The model under review builds one solid part; all positions refer to its coordinate system, in mm. Give positions to 0.01 mm unless a question says otherwise; leave off trailing zeros. Order: outer loops, then holes, each group sorted by start corner. A loop starts at its lowest first (then second) coordinate and runs counter-clockwise, first axis right, second up. Notation, with made-up numbers: (66.25, -26.75) -> (115.25, -26.75) arc R35 ccw to (115.25, 11.25) -> close; hole circle Ø1 at (58.5, 16.25). An arc over 180 degrees is marked (long way). Answer as a JSON object with one key per item and string values. Group by question number.
Autodesk Inventor part; units mm, degrees
ref_plane "YZ Plane" through (0, 0, 0) normal (1, 0, 0) x (0, 1, 0)
ref_plane "XZ Plane" through (0, 0, 0) normal (0, 1, 0) x (-1, 0, 0)
ref_plane "XY Plane" through (0, 0, 0) normal (0, 0, 1) x (1, 0, 0)
sketch "Sketch1" plane through (0, 0, 0) normal (0, 0, 1) x (1, 0, 0)
  circle A0 centre (0, 0) radius 9.525
  dimension "d0" = 19.05
extrude "Extrusion1" add sketch "Sketch1" along normal blind 3.175
sketch "Sketch2" plane through (0, 0, 3.175) normal (0, 0, 1) x (1, 0, 0)
  point P0 (0, 0)
  point P1 (0, 0)
hole "Hole1" at (0, 0, 3.175) direction (0, 0, -1) diameter 12.954 depth 25.4 tip angle 118
sketch "Sketch3" plane through (0, 0, 3.175) normal (0, 0, 1) x (1, 0, 0)
  point P0 (0, 0)
hole "Hole2" at (0, 0, 3.175) direction (0, 0, -1) diameter 13.208 depth 25.4 tip angle 118
properties part number "washer achobotics"
1. Take a section at D-D on y = -7.75. Give the boundary of the cut face in (x, z) (3 decimals).
2. For probe 1 along Y at (x, z) = (0, 1.7) (3 decimals); probe 2 along X at (y, z) = (-3.5, 0.5); probe 3 along X at (y, z) = (-2, 3), list the stretches that pass through material, from the lowest coordinate up. Write a range as [from, to].
3. Take a section at C-C on z = 0.85. Give the boundary of the cut face in (x, y) (3 decimals), plus the area to 3 significant figures.
4. For pin 1 (1.5 mm diameter, centred on x = -4.5, z = 1, fed in from -Y); pin 2 (10.5 mm diameter, centred on x = 0, y = 0, fed in from -Z), all flat-tipped, find the tip position at first contact; note any pin that passes through.
5. Draft analysis for pull direction Y (two halves, no side actions). For faces 1 (the cylindrical face through (2.53, -6.1, 1.57)), 2 (the flat face through (2, 6.5, 0)), 3 (the cylindrical face through (-7.559, 5.796, 1.565)), state which applies: pulls with the +Y half, pulls with the -Y half, needs draft (parallel to the pull), parting line crosses it, or undercut.
6. Take a section at A-A on y = 0. Give the boundary of the cut face in (x, z) (3 decimals).
Checks:
{
 "1": {"outline": "(-5.537, 0) -> (5.537, 0) -> (5.537, 3.175) -> (-5.537, 3.175) -> close"},
 "2": {"probe 1": "y = [-9.525, -6.604], [6.604, 9.525]", "probe 2": "x = [-8.86, -5.6], [5.6, 8.86]", "probe 3": "x = [-9.31, -6.29], [6.29, 9.31]"},
 "3": {"outline": "circle Ø19.05 at (0, 0); hole circle Ø13.208 at (0, 0)", "area": "148 mm2"},
 "4": {"pin 1": "stops at y = -8.76", "pin 2": "passes through"},
 "5": {"face 1": "undercut", "face 2": "needs draft", "face 3": "parting line crosses it"},
 "6": {"outline": "(-9.525, 0) -> (-6.604, 0) -> (-6.604, 3.175) -> (-9.525, 3.175) -> close; (6.604, 0) -> (9.525, 0) -> (9.525, 3.175) -> (6.604, 3.175) -> close"}
}
